Autodesk Inventor part; units mm, degrees
ref_plane "YZ Plane" through (0, 0, 0) normal (1, 0, 0) x (0, 1, 0)
ref_plane "XZ Plane" through (0, 0, 0) normal (0, 1, 0) x (-1, 0, 0)
ref_plane "XY Plane" through (0, 0, 0) normal (0, 0, 1) x (1, 0, 0)
sketch "Náčrt1" plane through (0, 0, 0) normal (0, 0, 1) x (1, 0, 0)
  line L0 (0, -50) -> (50, -50)
  line L1 (50, -50) -> (50, 50)
  line L2 (50, 50) -> (0, 50)
  line L3 (0, 50) -> (0, -50)
  point P0 (0, 0)
  point P1 (50, 0)
  point P2 (0, 0)
  dimension "d0" = 50
  dimension "d1" = 100
extrude "Vysunutí1" add sketch "Náčrt1" along normal blind 3
sketch "Náčrt2" plane through (50, -50, 0) normal (1, 0, 0) x (0, 0, -1)
  line L0 (0, 0) -> (0, 100)
  line L1 (0, 100) -> (-30, 86.0108)
  line L2 (-30, 86.0108) -> (-30, 83.804)
  line L3 (-30, 83.804) -> (0, 97.7932)
  line L4 (-3, 0) -> (-3, 100)
  line L5 (0, 100) -> (-3, 100)
  point P0 (0, 50)
  point P1 (-3, 98.6011)
  dimension "d4" = 65
  dimension "d6" = 2
  dimension "d7" = 30
extrude "Vysunutí2" add sketch "Náčrt2" against normal up to surface (50 mm away) contours L3 L4 L1 L0 | L3 L2 L1 L4
extrude "Vysunutí3" cut sketch "Náčrt2" against normal through all contours L1 L4 L5
ref_plane "Pracovní rovina1" through (50, 50, 0) normal (0, -1, 0) x (1, 0, 0)
sketch "Náčrt3" plane through (50, 50, 0) normal (0, -1, 0) x (1, 0, 0)
  line L0 (-14.865, 22.13) -> (-19.865, 22.13)
  line L1 (-19.865, 22.13) -> (-19.865, 13.2518)
  line L2 (-19.865, 13.2518) -> (-14.865, 13.2518)
  line L3 (-14.865, 13.2518) -> (-14.865, 22.13)
  line L4 (-50, 13.2518) -> (-45, 13.2518)
  line L5 (-45, 13.2518) -> (-45, 22.13)
  line L6 (-45, 22.13) -> (-50, 22.13)
  line L7 (-50, 22.13) -> (-50, 13.2518)
  line L8 (0, 0) -> (0, 30)
  line L9 (-50, 30) -> (-50, 0)
  line L10 (0, 0) -> (-50, 0)
  dimension "d12" = 5
  dimension "d13" = 22.13
  dimension "d14" = 25.135
properties part number "Test rampy"
Work out the finished part from the listing and answer in its coordinate system (mm). Round coordinates to 2 decimals unless told otherwise and drop trailing zeros. Loops run counter-clockwise (first coordinate to the right, second up) from the corner with the lowest first, then second, coordinate; pieces in that order, holes last. Notation, with made-up numbers: (64, -19.5) - (106, -19.5) arc R19 ccw to (106, -13.5) - close; hole circle Ø9 at (-39.75, 64). An arc over 180 degrees is marked (long way). Use one line per item in the form item = value. Start each with the question number.
(1) Find section C-C on z = 6.25. Determine the outline of the cut face in (x, y).
(2) Determine the mould class of faces 1 (the face through (25, 35, 30)), 2 (the face through (0, 8, 2)), 3 (the face through (25.35, 40.01, 16.69)) for opening direction Z: +Z half, -Z half, draft (parallel to the pull), parting line (faces both ways), or undercut.
(3) Consider line 1 (Z direction, x = 25, y = -1); line 2 (Z direction, x = 11.5, y = 38); line 3 (Y direction, x = 20, z = 21). Determine where each line is inside the solid, lowest interval first.
(4) Find section B-B on x = 42. Determine the outline of the cut face in (y, z), and give its area (3 significant figures).
(5) Flat-ended cylindrical pins translate along their axes: P1, Ø6, axis at x = 22, y = -16, coming from the -Z side; P2, Ø10, axis at x = 42.5, z = 11, coming from the -Y side; P3, Ø25, axis at x = 26.5, y = 8.5, coming from the +Z side; P4, Ø6, axis at x = 14.5, z = 9, coming from the -Y side. Find the tip coordinate at first contact, or state that the pin passes through.
(6) Find section A-A on y = -23.5. Determine the outline of the cut face in (x, z).
Answer list:
q1.outline = (0, 44.88) - (50, 44.88) - (50, 47.09) - (0, 47.09) - close
q2.face_1 = +Z half
q2.face_2 = draft
q2.face_3 = undercut
q3.line_1 = 0 to 3
q3.line_2 = 0 to 3, 21 to 25.73
q3.line_3 = 38 to 40.21
q4.outline = (-50, 0) - (50, 0) - (36.01, 30) - (33.8, 30) - (46.39, 3) - (-50, 3) - close
q4.area = 357 mm^2
q5.P1 = 0
q5.P2 = 40.33
q5.P3 = 3
q5.P4 = 42.2
q6.outline = (0, 0) - (50, 0) - (50, 3) - (0, 3) - close
